```python
from build123d import *

# Parameters (mm, degrees)
SKETCH_1_W                  = 10
SKETCH_1_H                  = 50
EXTRUDE_1_DEPTH             = 320
HOLE_WIZARD_2_D             = 6.6
HOLE_WIZARD_2_CBORE_D       = 11
HOLE_WIZARD_2_CBORE_DEPTH   = 6.8
HOLE_WIZARD_2_2_D           = 5.5
HOLE_WIZARD_2_2_CBORE_D     = 10
HOLE_WIZARD_2_2_CBORE_DEPTH = 5.7


with BuildPart() as part:
    # 草图1 → 凸台-拉伸1 (new body)
    with BuildSketch(Plane.XY):
        with Locations((5, 25)):
            Rectangle(SKETCH_1_W, SKETCH_1_H)
    extrude(amount=EXTRUDE_1_DEPTH)

    # Hole Wizard 2 (through all)
    with Locations(Plane(origin=(10, 7, 310), x_dir=(0, 0, 1), z_dir=(1, 0, 0))):
        with Locations((0, 0), (-150, 0), (-300, 0)):
            CounterBoreHole(HOLE_WIZARD_2_D / 2, HOLE_WIZARD_2_CBORE_D / 2, HOLE_WIZARD_2_CBORE_DEPTH)

    # Hole Wizard 2 2 (through all)
    with Locations(Plane(origin=(0, 37, 290), x_dir=(0, 0, -1), z_dir=(-1, 0, 0))):
        with Locations((0, 0), (0, 15), (260, 0), (260, 15)):
            CounterBoreHole(HOLE_WIZARD_2_2_D / 2, HOLE_WIZARD_2_2_CBORE_D / 2, HOLE_WIZARD_2_2_CBORE_DEPTH)


solid = part.part
```
Could you check a few things on this model? Use its own coordinates, in mm. A direction names the side the tool comes from. Give positions to 0.01 mm unless a question says otherwise; leave off trailing zeros. Write each loop counter-clockwise with the first axis right and the second up, starting at its lowest first coordinate (ties: lowest second). Pieces come first, ordered by that corner, then holes. Notation, with made-up numbers: (-20, 60.25) -> (31, 60.25) arc R14 ccw to (31, 73.25) -> close; hole circle Ø9 at (27, 9.25). An arc over 180 degrees is marked (long way). Write each question's results on one line, items separated by ' | '.
1. I want a section at B-B, the plane y = 37. Write out the boundary of the cut face in (x, z), then the cut area to 3 significant figures.
Check sheet entries:
outline: (0, 0) -> (10, 0) -> (10, 27.25) -> (5.7, 27.25) -> (5.7, 25) -> (0, 25) -> close; (0, 35) -> (5.7, 35) -> (5.7, 32.75) -> (10, 32.75) -> (10, 287.25) -> (5.7, 287.25) -> (5.7, 285) -> (0, 285) -> close; (0, 295) -> (5.7, 295) -> (5.7, 292.75) -> (10, 292.75) -> (10, 320) -> (0, 320) -> close | area: 3,040 mm²
2. I want a section at C-C, the plane z = 160. Write out the boundary of the cut face in (x, y).
Check sheet entries:
outline: (0, 0) -> (10, 0) -> (10, 1.5) -> (3.2, 1.5) -> (3.2, 3.7) -> (0, 3.7) -> close; (0, 10.3) -> (3.2, 10.3) -> (3.2, 12.5) -> (10, 12.5) -> (10, 50) -> (0, 50) -> close
3. I want a section at A-A, the plane z = 290. Write out the boundary of the cut face in (x, y).
Check sheet entries:
outline: (0, 0) -> (10, 0) -> (10, 19.25) -> (5.7, 19.25) -> (5.7, 17) -> (0, 17) -> close; (0, 27) -> (5.7, 27) -> (5.7, 24.75) -> (10, 24.75) -> (10, 34.25) -> (5.7, 34.25) -> (5.7, 32) -> (0, 32) -> close; (0, 42) -> (5.7, 42) -> (5.7, 39.75) -> (10, 39.75) -> (10, 50) -> (0, 50) -> close
4. On a 3-axis mill with a long thin cutter (end or side, diameter ignored), from which of +Z, -Z, +X, -X, +Y, -Y can I reach the whole of each face in a straight line? I mean faces 1 (the flat face through (5.7, 39.2, 27.8)), 2 (the cylindrical face through (7.88, 21.17, 292.62)), 3 (the flat face through (3.2, 7, 14)). Say none if no direction works.
Check sheet entries:
face 1: -X | face 2: +X, -X | face 3: +X
5. If we mould it in two halves opening along Z, with no side actions, what happens to faces 4 (the flat face through (5, 25, 0)), 5 (the flat face through (3.2, 11, 310)), 6 (the flat face through (0, 25, 158))? For each: released by +Z, released by -Z, zero draft, split by the parting line, or undercut.
Check sheet entries:
face 4: released by -Z | face 5: undercut | face 6: zero draft
6. I need wall thicknesses on L1, parallel to Z at x = 4.2, y = 37; L2, parallel to Y at x = 2.75, z = 30; L3, parallel to Y at x = 8.8, z = 290. Which ranges of each line are inside material? Lowest first, please.
Check sheet entries:
L1: z = 0 to 25, 35 to 285, 295 to 320 | L2: y = 0 to 17, 27 to 32, 42 to 50 | L3: y = 0 to 19.25, 24.75 to 34.25, 39.75 to 50
7. Will these pins go through, and if not, where does the flat tip stop? pin 1 Ø7 at (y, z) = (22, 290) entering from -X; pin 2 Ø4.5 at (y, z) = (37, 30) entering from -X.
Check sheet entries:
pin 1: stops at x = 5.7 | pin 2: passes through
